Model file for the job. Use its own axes, mm. Coordinates: 2 decimals unless noted, no trailing zeros. Loops run counter-clockwise (first coordinate to the right, second up) from the corner with the lowest first, then second, coordinate; pieces in that order, holes last.
from build123d import *

# Parameters (mm, degrees)
SKETCH1_W                      = 80.3
SKETCH1_H                      = 66
BOSS_EXTRUDE1_DEPTH            = 2
F_3_2_3_2_DIAMETER_HOLE1_D     = 3.2
FILLET1_R                      = 3
SKETCH4_W                      = 80.3
SKETCH4_H                      = 2
BOSS_EXTRUDE2_DEPTH            = 42
FILLET2_R                      = 20
F_3_2_3_2_DIAMETER_HOLE2_D     = 3.2
F_3_2_3_2_DIAMETER_HOLE2_DEPTH = 60
F_3_2_3_2_DIAMETER_HOLE2_TIP   = 0.96137699
SKETCH7_W                      = 75
SKETCH7_H                      = 60.5
CUT_EXTRUDE1_DEPTH             = 3
SKETCH10_W                     = 35
SKETCH10_H                     = 20
SKETCH10_W_2                   = 32
SKETCH10_H_2                   = 17
CUT_EXTRUDE3_DEPTH             = 3
SKETCH11_W                     = 75
SKETCH11_H                     = 0.25
CUT_EXTRUDE4_DEPTH             = 3


with BuildPart() as part:
    # Sketch1 → Boss-Extrude1 (new body)
    with BuildSketch(Plane.XY):
        with Locations((40.15, 33)):
            Rectangle(SKETCH1_W, SKETCH1_H)
    extrude(amount=BOSS_EXTRUDE1_DEPTH)

    # Ø3.2 (3.2) Diameter Hole1 (through all)
    with Locations(Plane.XY.offset(2)):
        with Locations((7, 59), (73.3, 59), (73.3, 7), (7, 7)):
            Hole(F_3_2_3_2_DIAMETER_HOLE1_D / 2)

    # Fillet1
    fillet1_edges = [part.edges().sort_by_distance(p)[0] for p in [
        (0, 66, 1),
        (80.3, 66, 1),
    ]]
    fillet(fillet1_edges, radius=FILLET1_R)

    # Sketch4 → Boss-Extrude2 (add)
    with BuildSketch(Plane.XZ):
        with Locations((40.15, 1)):
            Rectangle(SKETCH4_W, SKETCH4_H)
    extrude(amount=BOSS_EXTRUDE2_DEPTH)

    # Fillet2
    fillet2_edges = [part.edges().sort_by_distance(p)[0] for p in [
        (0, -42, 1),
        (80.3, -42, 1),
    ]]
    fillet(fillet2_edges, radius=FILLET2_R)

    # Ø3.2 (3.2) Diameter Hole2
    with Locations(Plane.XY.offset(2)):
        with Locations((7, -27), (73.3, -27)):
            Hole(F_3_2_3_2_DIAMETER_HOLE2_D / 2, depth=F_3_2_3_2_DIAMETER_HOLE2_DEPTH)
            with Locations((0, 0, -(F_3_2_3_2_DIAMETER_HOLE2_DEPTH + F_3_2_3_2_DIAMETER_HOLE2_TIP / 2))):  # 118° drill point
                Cone(0, F_3_2_3_2_DIAMETER_HOLE2_D / 2, F_3_2_3_2_DIAMETER_HOLE2_TIP, mode=Mode.SUBTRACT)

    # Sketch7 → Cut-Extrude1 (cut, through all)
    with BuildSketch(Plane.XY.offset(2)):
        with Locations((40.5, 33)):
            Rectangle(SKETCH7_W, SKETCH7_H)
    extrude(amount=-CUT_EXTRUDE1_DEPTH, mode=Mode.SUBTRACT)

    # Sketch10 → Cut-Extrude3 (cut, through all)
    with BuildSketch(Plane.XY.offset(2)):
        with Locations((21.5, -7.5)):
            Rectangle(SKETCH10_W, SKETCH10_H)
        Polygon((63.4, -17.5), (39, -17.5), (16.9, -17.5), (16.9, -38), (63.4, -38), align=None)
        with Locations((60.3, -6)):
            Rectangle(SKETCH10_W_2, SKETCH10_H_2)
    extrude(amount=-CUT_EXTRUDE3_DEPTH, mode=Mode.SUBTRACT)

    # Sketch11 → Cut-Extrude4 (cut, through all)
    with BuildSketch(Plane.XY.offset(2)):
        with Locations((40.5, 2.625)):
            Rectangle(SKETCH11_W, SKETCH11_H)
    extrude(amount=-CUT_EXTRUDE4_DEPTH, mode=Mode.SUBTRACT)


solid = part.part
Q1. Slice it at B-B (y = 50.5). List the corners of the cut face in (x, z), and give its area (3 significant figures).
Answers:
outline: (0, 0) - (3, 0) - (3, 2) - (0, 2) - close; (78, 0) - (80.3, 0) - (80.3, 2) - (78, 2) - close
area: 10.6 mm2
Q2. Drill centre lines: line 1 (Y direction, x = 19.5, z = 0.75); line 2 (Y direction, x = 73.3, z = 1.3); line 3 (X direction, y = 53, z = 1.45). Where is each one in solid material? Low to high.
Answers:
line 1: y = -41.99 to -38, 63.25 to 66
line 2: y = -37.2 to -28.6, -25.4 to -14.5, 63.25 to 66
line 3: x = 0 to 3, 78 to 80.3
Q3. Slice it at A-A (x = 55). List the corners of the cut face in (y, z), and give its area (3 significant figures).
Answers:
outline: (-42, 0) - (-38, 0) - (-38, 2) - (-42, 2) - close; (-17.5, 0) - (-14.5, 0) - (-14.5, 2) - (-17.5, 2) - close; (63.25, 0) - (66, 0) - (66, 2) - (63.25, 2) - close
area: 19.5 mm2
Q4. Slice it at C-C (x = 37.5). List the corners of the cut face in (y, z).
Answers:
outline: (-42, 0) - (-38, 0) - (-38, 2) - (-42, 2) - close; (63.25, 0) - (66, 0) - (66, 2) - (63.25, 2) - close
Q5. Slice it at D-D (z = 1.15). List the corners of the cut face in (x, y), and give its area (3 significant figures).
Answers:
outline: (0, -22) arc R20 ccw to (20, -42) - (60.3, -42) arc R20 ccw to (80.3, -22) - (80.3, 63) arc R3 ccw to (77.3, 66) - (3, 66) arc R3 ccw to (0, 63) - close; hole (3, 2.5) - (4, 2.5) - (4, -17.5) - (16.9, -17.5) - (16.9, -38) - (63.4, -38) - (63.4, -17.5) - (39, -17.5) - (39, 2.5) - (44.3, 2.5) - (44.3, -14.5) - (76.3, -14.5) - (76.3, 2.5) - (78, 2.5) - (78, 63.25) - (3, 63.25) - close; hole circle Ø3.2 at (7, -27); hole circle Ø3.2 at (73.3, -27)
area: 1,730 mm2
Q6. Flat gauge pin, fed straight in: P1, Ø10, axis at x = 31.5, y = -31, coming from the -Z side. Where does the tip first touch, or does it go through?
Answers:
P1: passes through
Q7. Mould opens along Y. For faces 1 (the cylindrical face through (74.597, -35.986, 1.014)), 2 (the cylindrical face through (7.208, -25.414, 0.986)), 3 (the flat face through (40, -4, 2)) say: +Y half, -Y half, draft (parallel to the pull), parting line (faces both ways), or undercut.
Answers:
face 1: -Y half
face 2: undercut
face 3: draft
